Answer from the drawing. Dimensions are ordinates in mm from the lowest x, y and z of the part. A direction names the side the tool comes from. Round coordinates to 2 decimals unless told otherwise and drop trailing zeros. Order: outer loops, then holes, each group sorted by start corner. A loop starts at its lowest first (then second) coordinate and runs counter-clockwise, first axis right, second up. Notation, with made-up numbers: M -5,17.5 L 20,17.5 A12 cw 20,27.5 Z; hole C 72.25,4 d7. An arc over 180 degrees is marked long. Answer as a JSON object with one key per item and string values. Group by question number.
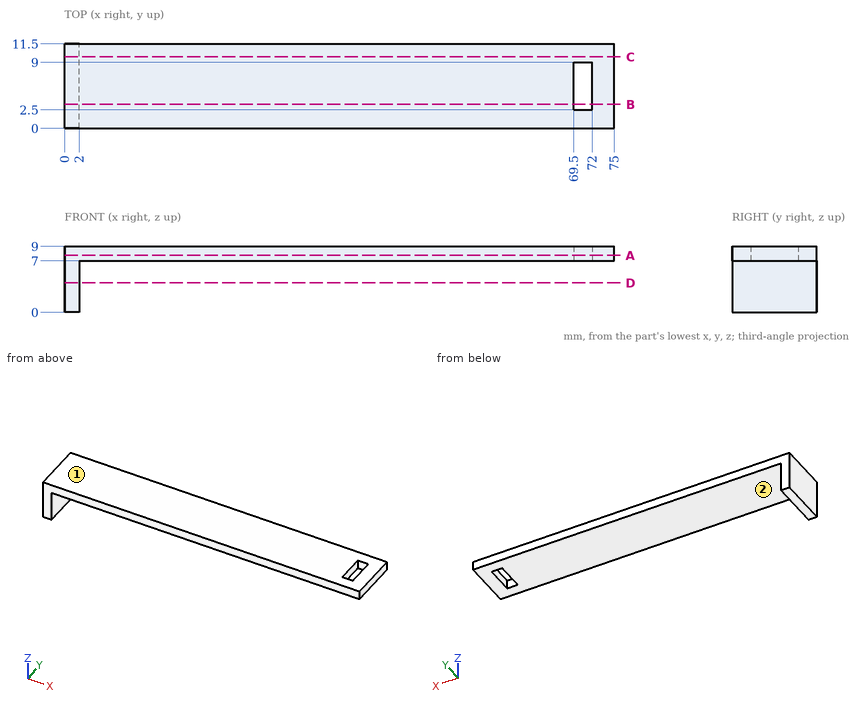
Item 1: Find section D-D (z = 4). Give the vertices of the cut face in (x, y), and give its area (3 significant figures).
Item 2: Find section A-A (z = 7.75). Give the vertices of the cut face in (x, y).
Item 3: A tool of negligible diameter and unlimited length cuts with its end or side. For the marked faces 1 and 2, from which of +Z, -Z, +X, -X, +Y, -Y can it reach the whole face along a straight path? Write none if from no direction.
Item 4: Find section C-C (y = 9.75). Give the vertices of the cut face in (x, z).
Item 5: Consider L1, parallel to X at y = 6, z = 1.5; L2, parallel to Z at x = 21.5, y = 6.5. Determine where each line is inside the solid, lowest interval first.
Item 6: This flat-tipped pin is pushed along its axis until it touches: pin 1 (3.5 mm diameter, centred on y = 7.5, z = 3, fed in from +X). Where does it stop, or does it pass through?
Item 7: Find section B-B (y = 3.25). Give the vertices of the cut face in (x, z), and give its area (3 significant figures).
Responses:
{
 "1": {"outline": "M 0,0 L 2,0 L 2,11.5 L 0,11.5 Z", "area": "23.0 mm^2"},
 "2": {"outline": "M 0,0 L 75,0 L 75,11.5 L 0,11.5 Z; hole M 69.5,2.5 L 72,2.5 L 72,9 L 69.5,9 Z"},
 "3": {"face 1": "+Z, +X, -X, +Y, -Y", "face 2": "-Z, +X, +Y, -Y"},
 "4": {"outline": "M 0,0 L 2,0 L 2,7 L 75,7 L 75,9 L 0,9 Z"},
 "5": {"L1": "x = 0 to 2", "L2": "z = 7 to 9"},
 "6": {"pin 1": "stops at x = 2"},
 "7": {"outline": "M 0,0 L 2,0 L 2,7 L 69.5,7 L 69.5,9 L 0,9 Z; M 72,7 L 75,7 L 75,9 L 72,9 Z", "area": "159 mm^2"}
}
